```python
from build123d import *

# Parameters (mm, degrees)
SKETCH1_W                 = 30
SKETCH1_H                 = 35
BOSS_EXTRUDE1_DEPTH       = 3
FILLET1_R                 = 10
SKETCH2_W                 = 10
SKETCH2_H                 = 3
CUT_EXTRUDE1_DEPTH        = 3
F_5_0MM_DOWEL_HOLE1_D     = 5
F_5_0MM_DOWEL_HOLE1_DEPTH = 3
F_5_0MM_DOWEL_HOLE1_TIP   = 1.502151548
CUT_EXTRUDE2_DEPTH        = 3
SKETCH6_W                 = 3
SKETCH6_H                 = 10
BOSS_EXTRUDE2_DEPTH       = 3


with BuildPart() as part:
    # Sketch1 → Boss-Extrude1 (new body)
    with BuildSketch(Plane(origin=(0, 0, 0), x_dir=(0, 0, -1), z_dir=(1, 0, 0))):
        with Locations((15, 17.5)):
            Rectangle(SKETCH1_W, SKETCH1_H)
    extrude(amount=BOSS_EXTRUDE1_DEPTH)

    # Fillet1
    fillet1_edges = [part.edges().sort_by_distance(p)[0] for p in [
        (1.5, 35, 0),
        (1.5, 35, -30),
    ]]
    fillet(fillet1_edges, radius=FILLET1_R)

    # Sketch2 → Cut-Extrude1 (cut)
    with BuildSketch(Plane(origin=(3, 0, 0), x_dir=(0, 0, -1), z_dir=(1, 0, 0))):
        with Locations((15, 1.5)):
            Rectangle(SKETCH2_W, SKETCH2_H)
    extrude(amount=-CUT_EXTRUDE1_DEPTH, mode=Mode.SUBTRACT)

    # Ø5.0mm Dowel Hole1
    with Locations(Plane(origin=(3, 0, 0), x_dir=(0, 0, -1), z_dir=(1, 0, 0))):
        with Locations((15, 20)):
            Hole(F_5_0MM_DOWEL_HOLE1_D / 2, depth=F_5_0MM_DOWEL_HOLE1_DEPTH)
            with Locations((0, 0, -(F_5_0MM_DOWEL_HOLE1_DEPTH + F_5_0MM_DOWEL_HOLE1_TIP / 2))):  # 118° drill point
                Cone(0, F_5_0MM_DOWEL_HOLE1_D / 2, F_5_0MM_DOWEL_HOLE1_TIP, mode=Mode.SUBTRACT)

    # Sketch5 → Cut-Extrude2 (cut)
    with BuildSketch(Plane(origin=(3, 0, 0), x_dir=(0, 0, -1), z_dir=(1, 0, 0))):
        Polygon((13.45, 3), (13.45, 6), (12.05, 6), (12.05, 8.7), (13.45, 8.7), (13.45, 10.3), (16.55, 10.3), (16.55, 8.7), (17.95, 8.7), (17.95, 6), (16.55, 6), (16.55, 3), align=None)
    extrude(amount=-CUT_EXTRUDE2_DEPTH, mode=Mode.SUBTRACT)

    # Sketch6 → Boss-Extrude2 (add)
    with BuildSketch(Plane(origin=(0, 35, 0), x_dir=(1, 0, 0), z_dir=(0, 1, 0))):
        with Locations((1.5, 15)):
            Rectangle(SKETCH6_W, SKETCH6_H)
    extrude(amount=BOSS_EXTRUDE2_DEPTH)


solid = part.part
```
Geometry: final body of the model. Coordinates: model frame, mm. A direction names the side the tool comes from. Round coordinates to 2 decimals unless told otherwise and drop trailing zeros. Write each loop counter-clockwise with the first axis right and the second up, starting at its lowest first coordinate (ties: lowest second). Pieces come first, ordered by that corner, then holes. Notation, with made-up numbers: M -24,15 L 7,15 A16 cw 7,24 Z; hole C 57,78.25 d10. An arc over 180 degrees is marked long. Answer in a Markdown table with one row per item. Add a question column.
(1) Ray query, L1, parallel to Y at x = 0.7, z = -15; L2, parallel to Z at x = 1.3, y = 20; L3, parallel to Z at x = 2.55, y = 4. Return the intervals inside material, ascending.
(2) Cut plane A-A, the plane y = 20. Return the cut outline in (x, z).
(3) Cut plane C-C, the plane x = 1.45. Return the cut outline in (y, z).
(4) Contact query for a flat-ended pin moving along its axis: pin 1 (1.1 mm diameter, centred on x = 2, z = -13, fed in from -Y). Output: stop coordinate, or through.
(5) Cut plane D-D, the plane z = -8.5. Return the cut outline in (x, y).
(6) Cut plane B-B, the plane z = -15. Return the cut outline in (x, y).
(7) Reachability of faces 1 (the face through (2, 9, -13.45)), 2 (the face through (1, 36, -10)), 3 (the face through (2, 6, -17)), 4 (the face through (1, 36, -20)), 5 (the face through (1, 12, 0)) from +Z, -Z, +X, -X, +Y, -Y: full face, straight path, thin tool, end or side. Return the list, or none.
(8) Draft query along Z for faces 6 (the face through (1, 12, -30)), 7 (the face through (1, 0, -5)), 8 (the face through (2, 5, -16.55)). Return one class per face: pulls with the +Z half, pulls with the -Z half, needs draft (parallel to the pull), parting line crosses it, or undercut.
Established:
| question | item | result |
|---|---|---|
| 1 | L1 | 10.3 to 17.5, 22.5 to 38 |
| 1 | L2 | -30 to -17.5, -12.5 to 0 |
| 1 | L3 | -30 to -16.55, -13.45 to 0 |
| 2 | outline | M 0,-30 L 3,-30 L 3,-17.5 L 0,-17.5 Z; M 0,-12.5 L 3,-12.5 L 3,0 L 0,0 Z |
| 3 | outline | M 0,-30 L 25,-30 A10 ccw 35,-20 L 38,-20 L 38,-10 L 35,-10 A10 ccw 25,0 L 0,0 L 0,-10 L 3,-10 L 3,-13.45 L 6,-13.45 L 6,-12.05 L 8.7,-12.05 L 8.7,-13.45 L 10.3,-13.45 L 10.3,-16.55 L 8.7,-16.55 L 8.7,-17.95 L 6,-17.95 L 6,-16.55 L 3,-16.55 L 3,-20 L 0,-20 Z; hole C 20,-15 d5 |
| 4 | pin 1 | y = 3 |
| 5 | outline | M 0,0 L 3,0 L 3,34.89 L 0,34.89 Z |
| 6 | outline | M 0,10.3 L 3,10.3 L 3,17.5 L 0,17.5 Z; M 0,22.5 L 3,22.5 L 3,38 L 0,38 Z |
| 7 | face 1 | +X, -X, -Y |
| 7 | face 2 | +Z, +X, -X, +Y |
| 7 | face 3 | +X, -X |
| 7 | face 4 | -Z, +X, -X, +Y |
| 7 | face 5 | +Z, +X, -X, +Y, -Y |
| 8 | face 6 | pulls with the -Z half |
| 8 | face 7 | needs draft |
| 8 | face 8 | undercut |
